Geometry: final body of the model. Coordinates: model frame, mm. A direction names the side the tool comes from. Round coordinates to 2 decimals unless told otherwise and drop trailing zeros. Order: outer loops, then holes, each group sorted by start corner. A loop starts at its lowest first (then second) coordinate and runs counter-clockwise, first axis right, second up. Notation, with made-up numbers: (5, 52.25) - (19, 52.25) arc R28 cw to (19, 80.25) - close; hole circle Ø9 at (53.5, -19.5). An arc over 180 degrees is marked (long way). Put each result on its own line as item: value. Start each with the question number.
(1) Section D-D (y = 3). Output: boundary loops of the cut face in (x, z), and give its area (3 significant figures).
(2) Access query for faces 1 (the face through (0, 2, 0)), 2 (the face through (0.325, 6.958, -8.536)). Directions: +Z, -Z, +X, -X, +Y, -Y. A direction counts if a zero-diameter tool reaches every point of the face in a straight line with its end or side. Return the directions, or none.
(3) Section C-C (z = 0). Output: boundary loops of the cut face in (x, y).
(4) Material intervals for L1, parallel to Z at x = 0, y = 8.15; L2, parallel to X at y = 6.5, z = 0; L3, parallel to Z at x = 1, y = 5.5, sorted ascending. Write a range as [from, to].
(5) Section A-A (z = -10). Output: boundary loops of the cut face in (x, y).
(6) Section B-B (x = 0). Output: boundary loops of the cut face in (y, z).
(7) Pin query (flat end, axial travel): P1, Ø6, axis at x = -3, z = 9, coming from the -Y side; P2, Ø2.5, axis at x = -1.5, z = 1.5, coming from the +Y side. Return the tip coordinate at first contact, or that it passes through.
(8) Pull-direction query (Z, two-part tool) for faces 3 (the face through (-0.943, 6.056, 4.247)), 4 (the face through (-4, 10, -3)); classes: released by +Z, released by -Z, zero draft, split by the parting line, or undercut.
Autodesk Inventor part; units mm, degrees
ref_plane "YZ Plane" through (0, 0, 0) normal (1, 0, 0) x (0, 1, 0)
ref_plane "XZ Plane" through (0, 0, 0) normal (0, 1, 0) x (-1, 0, 0)
ref_plane "XY Plane" through (0, 0, 0) normal (0, 0, 1) x (1, 0, 0)
sketch "Sketch1" plane through (0, 0, 0) normal (0, 1, 0) x (-1, 0, 0)
  circle A0 centre (0, 10) radius 1.5
  circle A1 centre (0, -10) radius 1.5
  arc A2 (2.6663, 8.625) -> (-2.6663, 8.625) centre (0, 10) ccw
  arc A3 (-2.6663, -8.625) -> (2.6663, -8.625) centre (0, -10) ccw
  arc A4 (2.6663, 8.625) -> (3.5551, 4.8333) centre (5.3327, 7.25) ccw
  arc A5 (-3.5551, 4.8333) -> (-2.6663, 8.625) centre (-5.3327, 7.25) ccw
  arc A6 (3.5551, -4.8333) -> (2.6663, -8.625) centre (5.3327, -7.25) ccw
  arc A7 (-2.6663, -8.625) -> (-3.5551, -4.8333) centre (-5.3327, -7.25) ccw
  arc A8 (-3.5551, 4.8333) -> (-3.5551, -4.8333) centre (0, 0) ccw
  arc A9 (3.5551, -4.8333) -> (3.5551, 4.8333) centre (0, 0) ccw
  dimension "d1" = 10
  dimension "d2" = 20
  dimension "d3" = 3
  dimension "d4" = 6
  dimension "d5" = 6
  dimension "d6" = 6
  dimension "d7" = 6
  dimension "d8" = 3
extrude "Extrusion1" add sketch "Sketch1" along normal blind 10
sketch "Sketch2" plane through (0, 10, 0) normal (0, 1, 0) x (1, 0, 0)
  circle A0 centre (0, 0) radius 4.35
  dimension "d11" = 8.7
extrude "Extrusion2" cut sketch "Sketch2" against normal blind 8
sketch "Sketch3" plane through (0, 0, 0) normal (0, -1, 0) x (1, 0, 0)
  circle A0 centre (0, 10) radius 1.5
  arc A1 (2.6663, 8.625) -> (-2.6663, 8.625) centre (0, 10) ccw
  circle A2 centre (0, -10) radius 1.5
  arc A3 (-2.6663, -8.625) -> (2.6663, -8.625) centre (0, -10) ccw
  arc A4 (2.6663, 8.625) -> (-2.6663, 8.625) centre (0, 10) ccw
  arc A5 (2.6663, 8.625) -> (3.5551, 4.8333) centre (5.3327, 7.25) ccw
  arc A6 (-3.5551, 4.8333) -> (-2.6663, 8.625) centre (-5.3327, 7.25) ccw
  arc A7 (-2.6663, -8.625) -> (-3.5551, -4.8333) centre (-5.3327, -7.25) ccw
  arc A8 (3.5551, -4.8333) -> (2.6663, -8.625) centre (5.3327, -7.25) ccw
  arc A9 (3.5551, -4.8333) -> (3.5551, 4.8333) centre (0, 0) ccw
  arc A10 (2.6663, 8.625) -> (3.5551, 4.8333) centre (5.3327, 7.25) ccw
  arc A11 (-3.5551, 4.8333) -> (-2.6663, 8.625) centre (-5.3327, 7.25) ccw
  arc A12 (-2.6663, -8.625) -> (-3.5551, -4.8333) centre (-5.3327, -7.25) ccw
  arc A13 (3.5551, -4.8333) -> (2.6663, -8.625) centre (5.3327, -7.25) ccw
  arc A14 (-3.5551, 4.8333) -> (-3.5551, -4.8333) centre (0, 0) ccw
  arc A15 (-2.6663, -8.625) -> (2.6663, -8.625) centre (0, -10) ccw
  arc A16 (3.5551, 4.8333) -> (-3.5551, 4.8333) centre (0, 0) ccw
  arc A17 (-3.5551, -4.8333) -> (3.5551, -4.8333) centre (0, 0) ccw
extrude "Extrusion3" cut sketch "Sketch3" against normal blind 4 contours A5 A16 A6 A1 | A8 A3 A7 A17
properties part number "Cap"
Checks:
1. outline: circle Ø12 at (0, 0); hole circle Ø8.7 at (0, 0)
1. area: 53.6 mm²
2. face 1: +Y
2. face 2: +Y, -Y
3. outline: (-6, 0) - (6, 0) - (6, 10) - (4.35, 10) - (4.35, 2) - (-4.35, 2) - (-4.35, 10) - (-6, 10) - close
4. L1: z = [-13, -11.5], [-8.5, -4.35], [4.35, 8.5], [11.5, 13]
4. L2: x = [-6, -4.35], [4.35, 6]
4. L3: z = [-12.83, -11.12], [-8.88, -4.23], [4.23, 8.88], [11.12, 12.83]
5. outline: (-3, 4) - (-1.5, 4) - (-1.5, 10) - (-3, 10) - close; (1.5, 4) - (3, 4) - (3, 10) - (1.5, 10) - close
6. outline: (0, -6) - (4, -6) - (4, -8.5) - (10, -8.5) - (10, -4.35) - (2, -4.35) - (2, 4.35) - (10, 4.35) - (10, 8.5) - (4, 8.5) - (4, 6) - (0, 6) - close; (4, -13) - (10, -13) - (10, -11.5) - (4, -11.5) - close; (4, 11.5) - (10, 11.5) - (10, 13) - (4, 13) - close
7. P1: stops at y = 4
7. P2: stops at y = 2
8. face 3: undercut
8. face 4: zero draft
